Autodesk Inventor part; units mm, degrees
ref_plane "YZ Plane" through (0, 0, 0) normal (1, 0, 0) x (0, 1, 0)
ref_plane "XZ Plane" through (0, 0, 0) normal (0, 1, 0) x (-1, 0, 0)
ref_plane "XY Plane" through (0, 0, 0) normal (0, 0, 1) x (1, 0, 0)
sketch "Sketch1" plane through (0, 0, 0) normal (0, 1, 0) x (-1, 0, 0)
  line L0 (-34.925, 6.35) -> (34.925, 6.35)
  line L1 (34.925, 6.35) -> (34.925, -6.35)
  line L2 (34.925, -6.35) -> (-34.925, -6.35)
  line L3 (-34.925, -6.35) -> (-34.925, 6.35)
  line L4 (-34.925, 6.35) -> (34.925, -6.35) construction
  line L5 (34.925, 6.35) -> (-34.925, -6.35) construction
  point P0 (0, 0)
  dimension "d0" = 69.85
  dimension "d1" = 12.7
extrude "Extrusion1" add sketch "Sketch1" along normal blind 12.7
sketch "Sketch2" plane through (-34.925, 0, -6.35) normal (-1, 0, 0) x (0, 0, 1)
  line L0 (0, 12.7) -> (12.7, 12.7)
  line L1 (3.2385, 0) -> (9.4615, 0)
  line L2 (9.4615, 0) -> (9.4615, 12.7)
  line L3 (9.4615, 12.7) -> (3.2385, 12.7)
  line L4 (3.2385, 12.7) -> (3.2385, 0)
  line L5 (3.2385, 0) -> (9.4615, 12.7) construction
  line L6 (9.4615, 0) -> (3.2385, 12.7) construction
  line L7 (12.7, 0) -> (12.7, 12.7)
  point P0 (6.35, 0)
  point P1 (6.35, 6.35)
  dimension "d4" = 6.223
  dimension "d5" = 12.7
  dimension "d6" = 3.2385
extrude "Extrusion2" add sketch "Sketch2" along normal blind 12.7
fillet "Fillet1" radius 10.16 1 edges at (-47.625, 0, 0)
sketch "Sketch3" plane through (-34.925, 0, 3.1115) normal (0, 0, 1) x (1, 0, 0)
  circle A0 centre (-6.35, 6.35) radius 3.175
  line L0 (0, 12.7) -> (-12.7, 12.7)
  line L1 (-12.7, 10.16) -> (-12.7, 12.7)
  point P0 (34.925, 0)
  dimension "d10" = 6.35
  dimension "d41" = 6.35
  dimension "d42" = 6.35
extrude "Extrusion3" cut sketch "Sketch3" against normal blind 12.7
sketch "Sketch4" plane through (0, 12.7, 0) normal (0, 1, 0) x (1, 0, 0)
  line L0 (-34.925, -3.1115) -> (-34.925, -6.35)
  line L1 (34.925, 6.35) -> (-34.925, 6.35)
  line L2 (-34.925, -6.35) -> (-22.225, -6.35)
  line L3 (-22.225, -6.35) -> (-22.225, 6.35)
  line L4 (-22.225, 6.35) -> (-34.925, 6.35)
  line L5 (-34.925, 6.35) -> (-34.925, -6.35)
  point P0 (0, 0)
  point P1 (-34.925, 6.35)
  dimension "d13" = 12.7
extrude "Extrusion4" add sketch "Sketch4" along normal blind 19.05
sketch "Sketch5" plane through (0, 31.75, 0) normal (0, 1, 0) x (1, 0, 0)
  line L0 (-34.925, -3.1115) -> (-34.925, -6.35)
  line L1 (-22.225, -6.35) -> (-22.225, 6.35)
  line L2 (-34.925, -3.175) -> (-22.225, -3.175)
  line L3 (-22.225, -3.175) -> (-22.225, 3.175)
  line L4 (-22.225, 3.175) -> (-34.925, 3.175)
  line L5 (-34.925, 3.175) -> (-34.925, -3.175)
  line L6 (-34.925, -6.35) -> (-22.225, -6.35)
  point P0 (0, 0)
  point P1 (-28.575, -6.35)
  dimension "d16" = 6.35
  dimension "d17" = 3.175
extrude "Extrusion5" cut sketch "Sketch5" against normal blind 12.7 contours L5 L4 L1 L2 L0
sketch "Sketch6" plane through (-34.925, 0, 6.35) normal (0, 0, 1) x (1, 0, 0)
  circle A0 centre (6.35, 25.4) radius 3.175
  line L0 (0, 31.75) -> (12.7, 31.75)
  line L1 (0, 0) -> (0, 31.75)
  point P0 (34.925, 0)
  dimension "d20" = 6.35
  dimension "d21" = 6.35
  dimension "d43" = 6.35
extrude "Extrusion6" cut sketch "Sketch6" against normal blind 12.7
sketch "Sketch7" plane through (0, 12.7, 0) normal (0, 1, 0) x (1, 0, 0)
  line L0 (34.925, -12.7) -> (9.525, -12.7)
  line L1 (9.525, -12.7) -> (9.525, 12.7)
  line L2 (9.525, 12.7) -> (34.925, 12.7)
  line L3 (34.925, 12.7) -> (34.925, -12.7)
  line L4 (34.925, -6.35) -> (34.925, 6.35)
  line L5 (-22.225, -6.35) -> (34.925, -6.35)
  point P0 (0, 0)
  dimension "d24" = 25.4
  dimension "d25" = 25.4
  dimension "d26" = 25.4
  dimension "d27" = 6.35
extrude "Extrusion7" add sketch "Sketch7" against normal blind 12.7
sketch "Sketch8" plane through (0, 0, 0) normal (0, -1, 0) x (1, 0, 0)
  circle A0 centre (22.225, 0) radius 8.89
  circle A1 centre (22.225, 0) radius 7.62
  line L0 (34.925, 12.7) -> (34.925, -12.7)
  point P0 (0, 0)
  dimension "d30" = 17.78
  dimension "d31" = 15.24
  dimension "d39" = 12.7
extrude "Extrusion8" add sketch "Sketch8" along normal blind 25.4
sketch "Sketch9" plane through (22.225, -25.4, 0) normal (0, -1, 0) x (1, 0, 0)
  circle A0 centre (0, 0) radius 6.2
  circle A1 centre (0, 0) radius 7.62
  point P0 (-22.225, 0)
  dimension "d34" = 12.4
  dimension "d45" = 15.24
extrude "Extrusion9" add sketch "Sketch9" against normal blind 2.54
sketch "Sketch10" plane through (22.225, 0, 0) normal (0, -1, 0) x (1, 0, 0)
  circle A0 centre (0, 0) radius 7.62
  point P0 (-22.225, 0)
extrude "Extrusion10" cut sketch "Sketch10" against normal blind 25.4
fillet "Fillet2" radius 7.62 2 edges at (-22.225, 31.75, 4.7625) (-22.225, 31.75, -4.7625)
properties part number "Press_Lower_Arm"
Work out the finished part from the listing and answer in its coordinate system (mm). A direction names the side the tool comes from. Coordinates: 2 decimals unless noted, no trailing zeros. Write each loop counter-clockwise with the first axis right and the second up, starting at its lowest first coordinate (ties: lowest second). Pieces come first, ordered by that corner, then holes.
Q1. A cutting plane is placed at C-C, the plane y = 6.35. State how many separate pieces and enclosed holes the cut face has, then the cut area to 3 significant figures.
Q2. A cutting plane is placed at D-D, the plane y = 25.4. Give the vertices of the cut face in (x, z) (3 decimals).
Q3. Determine the mould class of faces 4 (the face through (-44.447, 6.49, 0.044)), 5 (the face through (24.1, -25.4, 6.1)), 6 (the face through (-34.925, 16, 0)) for opening direction Y: released by +Y, released by -Y, zero draft, split by the parting line, or undercut.
Q4. Each of these flat-tipped pins is pushed along its axis until it touches: pin 1 Ø12 at (y, z) = (20, -5) entering from +X (3 decimals); pin 2 Ø4 at (y, z) = (15.5, -6.5) entering from -X (3 decimals); pin 3 Ø14.5 at (x, z) = (22.225, 0) entering from +Y. Where does it stop, or does it pass through?
Q5. Find the intervals of material crossed by line 1 (X direction, y = 7.5, z = 9.25) (3 decimals); line 2 (Y direction, x = 12, z = 11.25); line 3 (Y direction, x = 20, z = -8), in increasing order.
Q6. A cutting plane is placed at B-B, the plane x = 18. Give the vertices of the cut face in (y, z).
Q7. Which of the six approach directions +Z, -Z, +X, -X, +Y, -Y give full straight-line access (tool end or side, diameter ignored) to faces 1 (the face through (-29, 19.05, 0)), 2 (the face through (7, 12.7, 0)), 3 (the face through (-38, 8, 3.112))?
Q8. A cutting plane is placed at A-A, the plane z = 0. Give the vertices of the cut face in (x, y) (3 decimals).
Findings below:
1. separate pieces: 2
1. enclosed holes: 1
1. area: 1,060 mm2
2. outline: (-34.925, -6.35) - (-31.75, -6.35) - (-31.75, -3.175) - (-34.925, -3.175) - close; (-34.925, 3.175) - (-31.75, 3.175) - (-31.75, 6.35) - (-34.925, 6.35) - close; (-25.4, -6.35) - (-22.332, -6.35) - (-22.332, -3.175) - (-25.4, -3.175) - close; (-25.4, 3.175) - (-22.332, 3.175) - (-22.332, 6.35) - (-25.4, 6.35) - close
3. face 4: undercut
3. face 5: released by -Y
3. face 6: zero draft
4. pin 1: stops at x = -22.225
4. pin 2: stops at x = -34.925
4. pin 3: stops at y = -22.86
5. line 1: x = 9.525 to 34.925
5. line 2: y = 0 to 12.7
5. line 3: y = -25.4 to 12.7
6. outline: (-25.4, -7.82) - (0, -7.82) - (0, -12.7) - (12.7, -12.7) - (12.7, -6.34) - (-22.86, -6.34) - (-22.86, -4.54) - (-25.4, -4.54) - close; (-25.4, 4.54) - (-22.86, 4.54) - (-22.86, 6.34) - (12.7, 6.34) - (12.7, 12.7) - (0, 12.7) - (0, 7.82) - (-25.4, 7.82) - close
7. face 1: +X, -X, +Y
7. face 2: +Z, -Z, +X, +Y
7. face 3: +Z, -X, +Y, -Y
8. outline: (-47.625, 10.16) arc R10.16 ccw to (-37.465, 0) - (13.335, 0) - (13.335, -25.4) - (16.025, -25.4) - (16.025, -22.86) - (14.605, -22.86) - (14.605, 12.7) - (-22.225, 12.7) - (-22.225, 19.05) - (-34.925, 19.05) - (-34.925, 12.7) - (-47.625, 12.7) - close; (28.425, -25.4) - (31.115, -25.4) - (31.115, 0) - (34.925, 0) - (34.925, 12.7) - (29.845, 12.7) - (29.845, -22.86) - (28.425, -22.86) - close; hole circle Ø6.35 at (-41.275, 6.35)
